Check sheet for the drawn part. Datum: minimum x, y, z corner. Units: mm. A direction names the side the tool comes from. Round coordinates to 2 decimals unless told otherwise and drop trailing zeros. Loops run counter-clockwise (first coordinate to the right, second up) from the corner with the lowest first, then second, coordinate; pieces in that order, holes last. Notation, with made-up numbers: (-39, 67) - (-27, 67) arc R21 ccw to (-27, 76) - close; hole circle Ø2 at (81.25, 53.5). An arc over 180 degrees is marked (long way). Use CSV: the item, a comma, the result in double quotes.
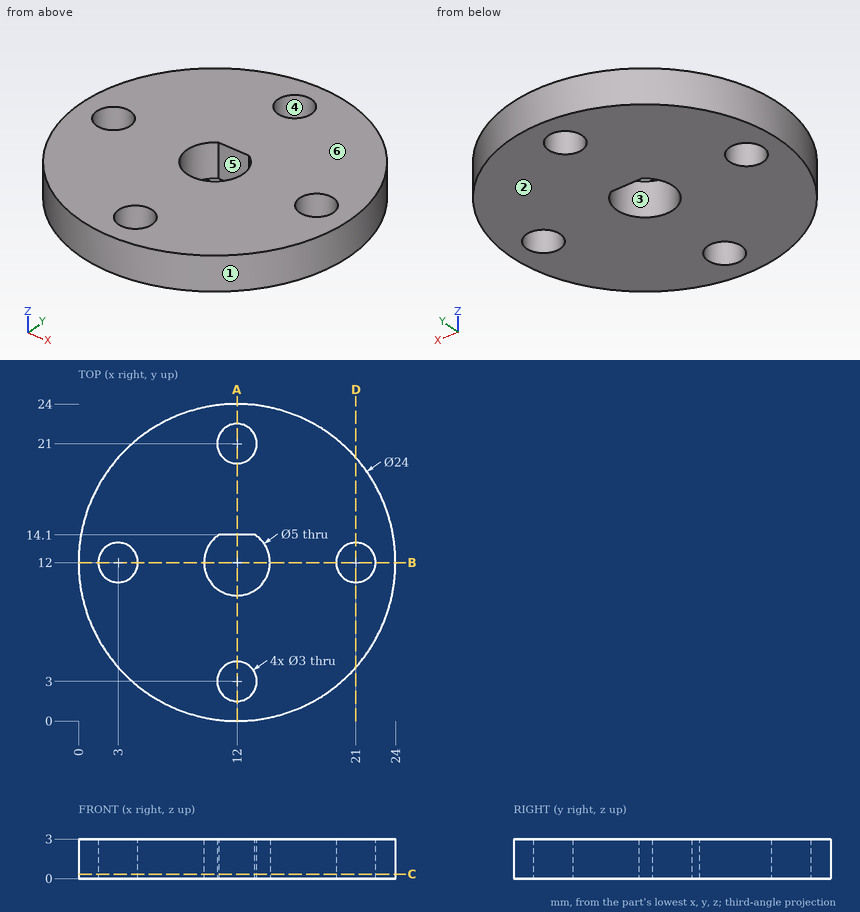
1) Thickness scan on probe 1 along Y at (x, z) = (12, 2.15); probe 2 along Y at (x, z) = (12.5, 1.45); probe 3 along X at (y, z) = (13.25, 2.05). Record the ranges inside material, lowest first. Write a range as [from, to].
Returned:
probe 1,"y = [0, 1.5], [4.5, 9.5], [14.1, 19.5], [22.5, 24]"
probe 2,"y = [0.01, 1.59], [4.41, 9.55], [14.1, 19.59], [22.41, 23.99]"
probe 3,"x = [0.07, 2.17], [3.83, 9.83], [14.17, 20.17], [21.83, 23.93]"
2) Cross-section at C-C, the plane z = 0.35. Record the cut outline in (x, y), then the cut area to 3 significant figures.
Returned:
outline,"circle Ø24 at (12, 12); hole circle Ø3 at (3, 12); hole circle Ø3 at (12, 3); hole circle Ø3 at (12, 21); hole (10.64, 14.1) arc R2.5 ccw (long way) to (13.36, 14.1) - close; hole circle Ø3 at (21, 12)"
area,"405 mm²"
3) Cross-section at D-D, the plane x = 21. Record the cut outline in (y, z).
Returned:
outline,"(4.06, 0) - (10.5, 0) - (10.5, 3) - (4.06, 3) - close; (13.5, 0) - (19.94, 0) - (19.94, 3) - (13.5, 3) - close"
4) Access from +Z, -Z, +X, -X, +Y, -Y to the whole of each face (thin tool, end or side, straight path). Record for the marked faces 5 and 6.
Returned:
face 5,"+Z, -Z"
face 6,"+Z, +X, -X, +Y, -Y"
5) Gauge pin test, flat ends, axial feed: pin 1 Ø1 at (x, y) = (13, 13.5) entering from -Z; pin 2 Ø1.5 at (y, z) = (4.5, 2.5) entering from +X. Record the tip position at first contact, or that the pin passes through.
Returned:
pin 1,"passes through"
pin 2,"stops at x = 21.92"
6) Cross-section at A-A, the plane x = 12. Record the cut outline in (y, z).
Returned:
outline,"(0, 0) - (1.5, 0) - (1.5, 3) - (0, 3) - close; (4.5, 0) - (9.5, 0) - (9.5, 3) - (4.5, 3) - close; (14.1, 0) - (19.5, 0) - (19.5, 3) - (14.1, 3) - close; (22.5, 0) - (24, 0) - (24, 3) - (22.5, 3) - close"
7) Mould release check, pull along X, two halves, no side actions. Record for the marked faces 1, 2, 3 and 4: +X half, -X half, draft (parallel to the pull), parting line (faces both ways), or undercut.
Returned:
face 1,"parting line"
face 2,"draft"
face 3,"undercut"
face 4,"undercut"
8) Cross-section at B-B, the plane y = 12. Record the cut outline in (x, z), then the cut area to 3 significant figures.
Returned:
outline,"(0, 0) - (1.5, 0) - (1.5, 3) - (0, 3) - close; (4.5, 0) - (9.5, 0) - (9.5, 3) - (4.5, 3) - close; (14.5, 0) - (19.5, 0) - (19.5, 3) - (14.5, 3) - close; (22.5, 0) - (24, 0) - (24, 3) - (22.5, 3) - close"
area,"39.0 mm²"
